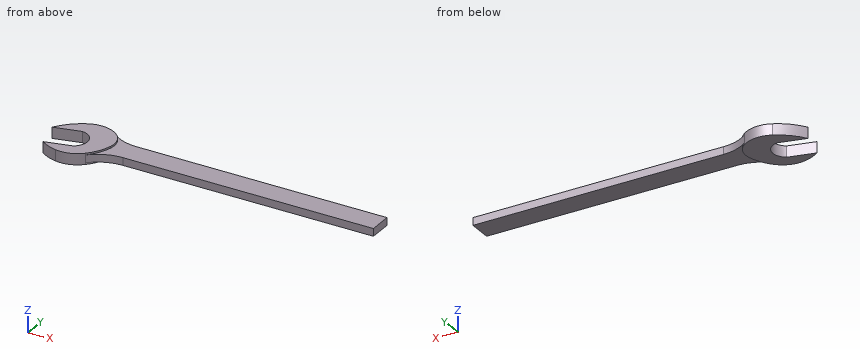
from build123d import *

# Parameters (mm, degrees)
PAD_DEPTH    = 2.65
PAD001_DEPTH = 3.85


with BuildPart() as part:
    # Sketch001 → Pad (new body, symmetric)
    with BuildSketch(Plane.XY):
        with BuildLine():
            ThreePointArc((-18, 31.032135), (-9.486833, 26.571636), (0, 25.032135))
            Line((0, 25.032135), (140, 25.032135))
            Line((140, 25.032135), (175, 25.032135))
            Line((175, 25.032135), (175, 9.032135))
            Line((140, 9.032135), (175, 9.032135))
            Line((0, 9.032135), (140, 9.032135))
            ThreePointArc((0, 9.032135), (-11.341769, 6.80558), (-21, 0.45642))
            ThreePointArc((-21, 0.45642), (-15.685703, 7.338058), (-12.444835, 15.406233))
            ThreePointArc((-12.444835, 15.406233), (-12.866577, 24.056709), (-18, 31.032135))
        make_face()
    extrude(amount=PAD_DEPTH, both=True)

    # Sketch → Pad001 (join, symmetric)
    with BuildSketch(Plane.XY):
        with BuildLine():
            Line((-55, 18.435619), (-36.564381, 23.032135))
            ThreePointArc((-31.967865, 4.596516), (-27.592913, 15.478143), (-36.564381, 23.032135))
            Line((-50.403484, 0), (-31.967865, 4.596516))
            ThreePointArc((-50.403484, 0), (-44.770144, -3.102558), (-38.604972, -4.933145))
            ThreePointArc((-38.604972, -4.933145), (-29.145429, -4.384635), (-21, 0.45642))
            ThreePointArc((-21, 0.45642), (-15.685703, 7.338058), (-12.444835, 15.406233))
            ThreePointArc((-12.444835, 15.406233), (-12.866577, 24.056709), (-18, 31.032135))
            ThreePointArc((-18, 31.032135), (-28.137567, 34.94523), (-38.824935, 32.979851))
            ThreePointArc((-38.824935, 32.979851), (-47.920113, 26.828366), (-55, 18.435619))
        make_face()
    extrude(amount=PAD001_DEPTH, both=True)


solid = part.part
Here's how the part is built. I have some questions about the finished solid (model axes, mm). Coordinates: 2 decimals unless noted, no trailing zeros. Order: outer loops, then holes, each group sorted by start corner. A loop starts at its lowest first (then second) coordinate and runs counter-clockwise, first axis right, second up. Notation, with made-up numbers: (63.5, 33) -> (119.5, 33) arc R15 ccw to (119.5, 55) -> close; hole circle Ø5 at (23, -12). An arc over 180 degrees is marked (long way). Answer in a Markdown table with one row per item.
(1) I want a section at A-A on z = 0.25. List the corners of the cut face in (x, y) for me.
Answer key:
| item | result |
|---|---|
| outline | (-55, 18.44) -> (-36.56, 23.03) arc R10 cw to (-31.97, 4.6) -> (-50.4, 0) arc R30 ccw to (-38.6, -4.93) arc R20 ccw to (-21, 0.46) arc R30 cw to (0, 9.03) -> (175, 9.03) -> (175, 25.03) -> (0, 25.03) arc R30 cw to (-18, 31.03) arc R20 ccw to (-38.82, 32.98) arc R40 ccw to start |
(2) I want a section at B-B on y = 27. List the corners of the cut face in (x, z) for me.
Answer key:
| item | result |
|---|---|
| outline | (-47.73, -3.85) -> (-14.29, -3.85) -> (-14.29, -2.65) -> (-10.69, -2.65) -> (-10.69, 2.65) -> (-14.29, 2.65) -> (-14.29, 3.85) -> (-47.73, 3.85) -> close |
(3) I want a section at C-C on x = 12.5. List the corners of the cut face in (y, z) for me, then the cut area to 3 significant figures.
Answer key:
| item | result |
|---|---|
| outline | (9.03, -2.65) -> (25.03, -2.65) -> (25.03, 2.65) -> (9.03, 2.65) -> close |
| area | 84.8 mm^2 |
(4) Will these pins go through, and if not, where does the flat tip stop? pin 1 Ø1.5 at (y, z) = (10.5, 0) entering from -X; pin 2 Ø1.5 at (x, y) = (120, 26) entering from +Z; pin 3 Ø5 at (x, y) = (105, 18.5) entering from -Z; pin 4 Ø2.5 at (x, z) = (128.5, -0.5) entering from +Y.
Answer key:
| item | result |
|---|---|
| pin 1 | x = -27.86 |
| pin 2 | through |
| pin 3 | z = -2.65 |
| pin 4 | y = 25.03 |
(5) Please list where these lines run through material, in increasing order: probe 1 along Y at (x, z) = (50, 1.75); probe 2 along Z at (x, y) = (154.5, 11.5); probe 3 along Y at (x, z) = (-44.5, -2).
Answer key:
| item | result |
|---|---|
| probe 1 | 9.03 to 25.03 |
| probe 2 | -2.65 to 2.65 |
| probe 3 | -3.21 to 1.47, 21.05 to 29.58 |
